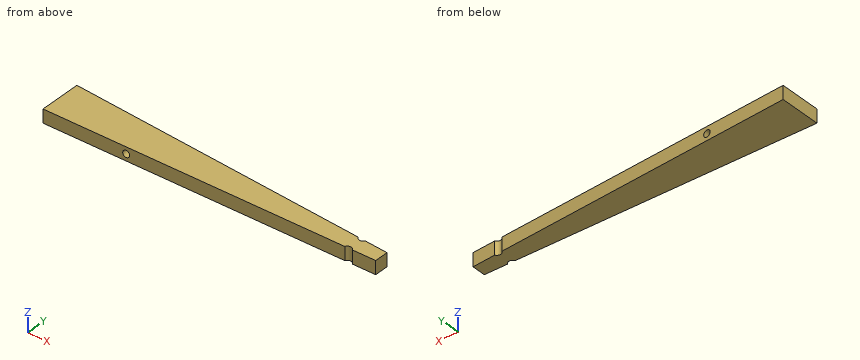
```python
from build123d import *

# Parameters (mm, degrees)
F1_DEPTH = 12.7
F3_DEPTH = 25.4
F5_DEPTH = 50.8


with BuildPart() as f1:
    # F0 (on Top) → F1 (new body)
    with BuildSketch(Plane.XY):
        Polygon((221.4371956441, 15.4739474714), (-83.0981060863, 28.1739474714), (-83.0981060863, -9.9260525286), (221.4371956441, 2.7739474714), align=None)
    extrude(amount=F1_DEPTH)

    # F2 (on face) → F3 (cut)
    with BuildSketch(Plane.XY.offset(12.7)):
        with BuildLine():
            Line((200.0921744873, 16.3640963873), (193.1399459127, 16.6540243608))
            ThreePointArc((193.1399459127, 16.6540243608), (196.5220172711, 14.2539901577), (200.0921744873, 16.3640963873))
        make_face()
        with BuildLine():
            ThreePointArc((200.0921744873, 1.8837985555), (196.5220172711, 3.9939047851), (193.1399459127, 1.5938705819))
            Line((193.1399459127, 1.5938705819), (200.0921744873, 1.8837985555))
        make_face()
    extrude(amount=-F3_DEPTH, mode=Mode.SUBTRACT)

    # F4 (on face) → F5 (cut)
    with BuildSketch(Plane(origin=(0.2689588056, -6.4494055911, 0), x_dir=(0.9991315674, 0.0416666667, 0), z_dir=(0.0416666667, -0.9991315674, 0))):
        with BuildLine():
            ThreePointArc((-4.0645265004, 6.35), (-7.2395265004, 9.525), (-10.4145265004, 6.35))
            ThreePointArc((-10.4145265004, 6.35), (-7.2395265004, 3.175), (-4.0645265004, 6.35))
        make_face()
    extrude(amount=-F5_DEPTH, mode=Mode.SUBTRACT)


solid = f1.part
```
CAD build for the part. Positions are in the model's coordinates, mm. Coordinates: 2 decimals unless noted, no trailing zeros. Order: outer loops, then holes, each group sorted by start corner. A loop starts at its lowest first (then second) coordinate and runs counter-clockwise, first axis right, second up. Notation, with made-up numbers: (5, -31) -> (17, -31) arc R21 cw to (17, -24) -> close; hole circle Ø2 at (58.25, -32). An arc over 180 degrees is marked (long way). Use one line per item in the form item = value. Start each with the question number.
1) Drill centre lines: L1, parallel to Y at x = 173, z = 6.75; L2, parallel to Y at x = 5, z = 4.25. Where is each one in solid material? Low to high. Write a range as [from, to].
2) Band-saw the part on B-B on x = 160.5. Give the cut face in (y, z).
3) Drop a flat-ended pin along its axis: pin 1 (5 mm diameter, centred on x = 55, z = 5.5, fed in from +Y). Give the stop position or say it passes through.
4) Band-saw the part on A-A on x = -32.5. Give the cut face in (y, z), then the cut area to 3 significant figures.
Entries:
q1.L1 = [0.75, 17.49]
q1.L2 = [-6.25, 24.5]
q2.outline = (0.23, 0) -> (18.02, 0) -> (18.02, 12.7) -> (0.23, 12.7) -> close
q3.pin_1 = 22.52
q4.outline = (-7.82, 0) -> (26.06, 0) -> (26.06, 12.7) -> (-7.82, 12.7) -> close
q4.area = 430 mm2
